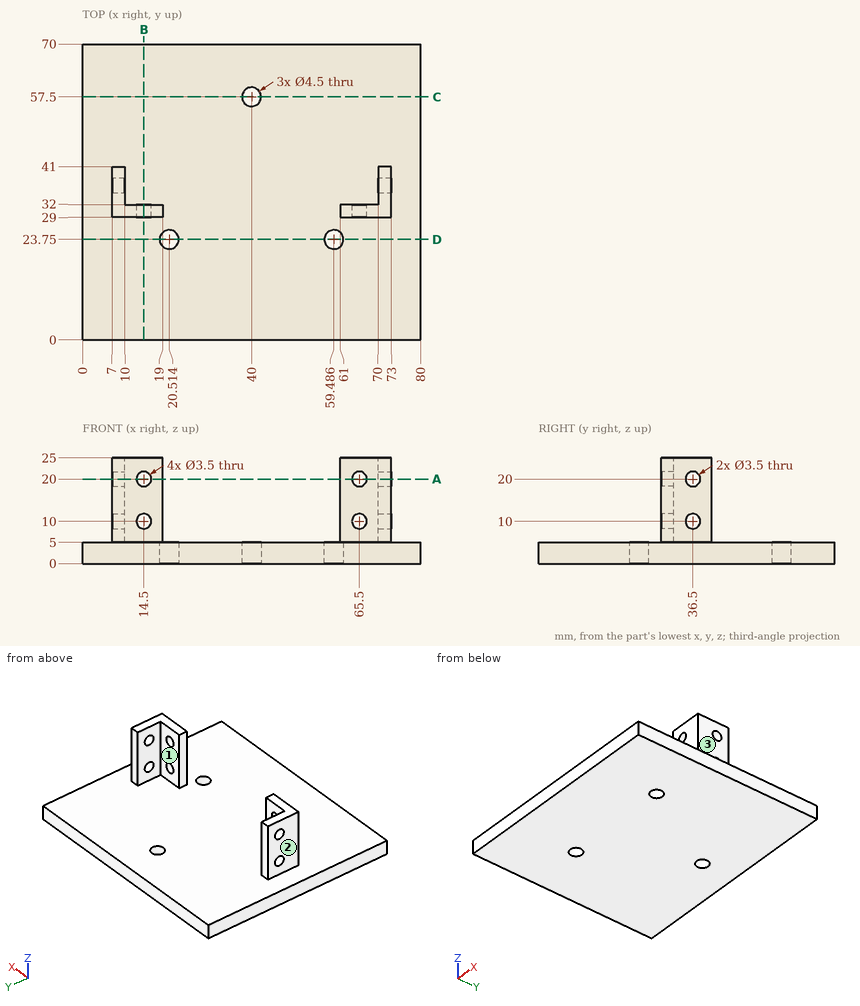
Job drawing, mm, ordinate dimensions from the low corner. One solid piece. A direction names the side the tool comes from. Give positions to 0.01 mm unless a question says otherwise; leave off trailing zeros. Order: outer loops, then holes, each group sorted by start corner. A loop starts at its lowest first (then second) coordinate and runs counter-clockwise, first axis right, second up. Notation, with made-up numbers: M -3,-38.75 L 28,-38.75 A16 ccw 28,-28.75 Z; hole C -26,11.25 d7. An arc over 180 degrees is marked long. Return JSON: item names as keys, results as strings.
Q1. 3-axis set-ups, long thin cutter, end or side, ignore diameter. For the marked faces 1, 2 and 3: which of +Z, -Z, +X, -X, +Y, -Y reach the whole face in a straight line?
Answer list:
{"face 1": "+Z, +Y", "face 2": "+Z, -X, +Y, -Y", "face 3": "+Z, +X, +Y, -Y"}
Q2. Band-saw the part on A-A (z = 20). Give the cut face in (x, y).
Answer list:
{"outline": "M 7,29 L 12.75,29 L 12.75,32 L 10,32 L 10,34.75 L 7,34.75 Z; M 7,38.25 L 10,38.25 L 10,41 L 7,41 Z; M 16.25,29 L 19,29 L 19,32 L 16.25,32 Z; M 61,29 L 63.75,29 L 63.75,32 L 61,32 Z; M 67.25,29 L 73,29 L 73,34.75 L 70,34.75 L 70,32 L 67.25,32 Z; M 70,38.25 L 73,38.25 L 73,41 L 70,41 Z"}
Q3. Flat gauge pins, fed straight in: pin 1 (3.5 mm diameter, centred on y = 36, z = 19.5, fed in from -X); pin 2 (7 mm diameter, centred on x = 20.51, y = 23.75, fed in from +Z); pin 3 (5 mm diameter, centred on y = 14, z = 6, fed in from +X); pin 4 (3.5 mm diameter, centred on x = 72, z = 10.5, fed in from +Y). Where does each tip first touch, or does it go through?
Answer list:
{"pin 1": "stops at x = 7", "pin 2": "stops at z = 5", "pin 3": "stops at x = 80", "pin 4": "stops at y = 41"}
Q4. Band-saw the part on D-D (y = 23.75). Give the cut face in (x, z) (1 decimal).
Answer list:
{"outline": "M 0,0 L 18.3,0 L 18.3,5 L 0,5 Z; M 22.8,0 L 57.2,0 L 57.2,5 L 22.8,5 Z; M 61.7,0 L 80,0 L 80,5 L 61.7,5 Z"}
Q5. Band-saw the part on C-C (y = 57.5). Give the cut face in (x, z).
Answer list:
{"outline": "M 0,0 L 37.75,0 L 37.75,5 L 0,5 Z; M 42.25,0 L 80,0 L 80,5 L 42.25,5 Z"}
Q6. Wall check: probe 1 along Z at (x, y) = (8.8, 36.5); probe 2 along Y at (x, z) = (12.5, 23); probe 3 along Z at (x, y) = (55.5, 67). Give the ranges that are in metal, low to high. Write a range as from..to.
Answer list:
{"probe 1": "z = 0..8.25, 11.75..18.25, 21.75..25", "probe 2": "y = 29..32", "probe 3": "z = 0..5"}
Q7. Band-saw the part on B-B (x = 14.5). Give the cut face in (y, z), then the cut area to 3 significant figures.
Answer list:
{"outline": "M 0,0 L 70,0 L 70,5 L 32,5 L 32,8.25 L 29,8.25 L 29,5 L 0,5 Z; M 29,11.75 L 32,11.75 L 32,18.25 L 29,18.25 Z; M 29,21.75 L 32,21.75 L 32,25 L 29,25 Z", "area": "389 mm^2"}
